The model under review builds one solid part; all positions refer to its coordinate system, in mm. A direction names the side the tool comes from. Coordinates: 2 decimals unless noted, no trailing zeros. Write each loop counter-clockwise with the first axis right and the second up, starting at its lowest first coordinate (ties: lowest second). Pieces come first, ordered by that corner, then holes.
1) Machinability: for faces 4 (the flat face through (39.55, 0, -8)), 5 (the flat face through (44, 0, -7)), 6 (the cylindrical face through (-41.685, -24.919, 3.979)), 7 (the flat face through (-39, 26, 5.5)), 8 (the cylindrical face through (54.05, -25.38, -3.09)), which of the approach directions +Z, -Z, +X, -X, +Y, -Y give a long, thin tool a straight path to every point of the face, cutting with its end or side? Answer none if there is none.
2) Add section B-B, the plane z = 4.5. State the section outline as (x, y) points, then the cut area to 3 significant figures.
3) Add section C-C, the plane z = -8. State the section outline as (x, y) points.
4) For P1, Ø8, axis at x = -22, y = 20, coming from the -Z side; P2, Ø3, axis at x = 51, z = -4.5, coming from the -Y side; P3, Ø8, axis at x = 14.5, z = -7, coming from the +Y side; P4, Ø2.5, axis at x = -43, y = -6, coming from the +Z side, all flat-tipped, find the tip position at first contact; note any pin that passes through.
5) Add section A-A, the plane x = 43.32. Give the number of separate pieces and of enclosed holes in the cut face, then the cut area to 3 significant figures.
6) Add section D-D, the plane y = -9.5. State the section outline as (x, z) points.
7) Mouldability with a two-part tool opening along X and no side actions: class faces 1 (the flat face through (-47, 0, -9.5)), 2 (the cylindrical face through (-41.609, 25.126, 3.979)), 3 (the flat face through (54.3, 0, -3)) as released by +X, released by -X, zero draft, split by the parting line, or undercut.
8) For line 1 (X direction, y = -25.5, z = -3.5) (3 decimals); line 2 (X direction, y = 13, z = -1.25); line 3 (Y direction, x = -39.3, z = 3.1), list the stretches that pass through material, from the lowest coordinate up.
from build123d import *

# Parameters (mm, degrees)
SKETCH1_W            = 108.6
SKETCH1_H            = 53.4162
BOSS_EXTRUDE1_DEPTH  = 2.5
SKETCH2_R            = 2.5
BOSS_EXTRUDE2_DEPTH  = 3
M3_CLEARANCE_HOLE1_D = 3.2
SKETCH5_W            = 6.75
SKETCH5_H            = 53.4162
BOSS_EXTRUDE3_DEPTH  = 9.5
SKETCH6_W            = 2.5
SKETCH6_H            = 53.4162
BOSS_EXTRUDE4_DEPTH  = 8
SKETCH7_W            = 2.5
SKETCH7_H            = 53.4162
BOSS_EXTRUDE5_DEPTH  = 8
SKETCH8_R            = 3.15
CUT_EXTRUDE1_DEPTH   = 2.7


with BuildPart() as part:
    # Sketch1 → Boss-Extrude1 (new body)
    with BuildSketch(Plane.XY):
        Rectangle(SKETCH1_W, SKETCH1_H)
    extrude(amount=BOSS_EXTRUDE1_DEPTH)

    # Sketch2 → Boss-Extrude2 (add)
    with BuildSketch(Plane.XY.offset(2.5)):
        with Locations(Location((-39.3, 24.1681, 0), (0, 0, 180))):
            Circle(SKETCH2_R)
        with Locations(Location((35.83, 24.1681, 0), (0, 0, 180))):
            Circle(SKETCH2_R)
        with Locations(Location((43.32, -24.16810902, 0), (0, 0, 180))):
            Circle(SKETCH2_R)
        with Locations(Location((-39.3, -24.16810902, 0), (0, 0, 180))):
            Circle(SKETCH2_R)
    extrude(amount=BOSS_EXTRUDE2_DEPTH)

    # M3 Clearance Hole1 (through all)
    with Locations(Plane.XY.offset(5.5)):
        with Locations((-39.3, 24.1681), (35.83, 24.1681), (43.32, -24.16810902), (-39.3, -24.16810902)):
            Hole(M3_CLEARANCE_HOLE1_D / 2)

    # Sketch5 → Boss-Extrude3 (add)
    with BuildSketch(Plane(origin=(0, 0, 0), x_dir=(-1, 0, 0), z_dir=(0, 0, -1))):
        with Locations((-50.925, 0)):
            Rectangle(SKETCH5_W, SKETCH5_H)
        with Locations((50.925, 0)):
            Rectangle(SKETCH5_W, SKETCH5_H)
    extrude(amount=BOSS_EXTRUDE3_DEPTH)

    # Sketch6 → Boss-Extrude4 (add)
    with BuildSketch(Plane.ZY.offset(-47.55)):
        with Locations((-8.25, 0)):
            Rectangle(SKETCH6_W, SKETCH6_H)
    extrude(amount=BOSS_EXTRUDE4_DEPTH)

    # Sketch7 → Boss-Extrude5 (add)
    with BuildSketch(Plane(origin=(-47.55, 0, 0), x_dir=(0, 0, -1), z_dir=(1, 0, 0))):
        with Locations((8.25, 0)):
            Rectangle(SKETCH7_W, SKETCH7_H)
    extrude(amount=BOSS_EXTRUDE5_DEPTH)

    # Sketch8 → Cut-Extrude1 (cut)
    with BuildSketch(Plane.XZ.offset(26.7081)):
        with Locations(Location((-50.925, -3.5, 0), (0, 0, 270))):
            Circle(SKETCH8_R)
        with Locations(Location((50.925, -3.5, 0), (0, 0, 270))):
            Circle(SKETCH8_R)
    extrude(amount=-CUT_EXTRUDE1_DEPTH, mode=Mode.SUBTRACT)


solid = part.part
Geometry results:
1. face 4: -Z, +Y, -Y
1. face 5: +Y, -Y
1. face 6: +Z
1. face 7: +Z, +X, -X, +Y, -Y
1. face 8: -Y
2. outline: circle Ø5 at (-39.3, -24.17); circle Ø5 at (-39.3, 24.17); circle Ø5 at (35.83, 24.17); circle Ø5 at (43.32, -24.17); hole circle Ø3.2 at (-39.3, -24.17); hole circle Ø3.2 at (-39.3, 24.17); hole circle Ø3.2 at (35.83, 24.17); hole circle Ø3.2 at (43.32, -24.17)
2. area: 46.4 mm2
3. outline: (-54.3, -26.71) - (-39.55, -26.71) - (-39.55, 26.71) - (-54.3, 26.71) - close; (39.55, -26.71) - (54.3, -26.71) - (54.3, 26.71) - (39.55, 26.71) - close
4. P1: stops at z = 0
4. P2: stops at y = -24.01
4. P3: passes through
4. P4: stops at z = 2.5
5. separate pieces: 3
5. enclosed holes: 0
5. area: 264 mm2
6. outline: (-54.3, -9.5) - (-39.55, -9.5) - (-39.55, -7) - (-47.55, -7) - (-47.55, 0) - (47.55, 0) - (47.55, -7) - (39.55, -7) - (39.55, -9.5) - (54.3, -9.5) - (54.3, 2.5) - (-54.3, 2.5) - close
7. face 1: zero draft
7. face 2: undercut
7. face 3: released by +X
8. line 1: x = -54.3 to -54.075, -47.775 to -47.55, 47.55 to 47.775, 54.075 to 54.3
8. line 2: x = -54.3 to -47.55, 47.55 to 54.3
8. line 3: y = -26.67 to -25.77, -22.57 to -21.67, 21.67 to 22.57, 25.77 to 26.67
